```python
from build123d import *

# Parameters (mm, degrees)
SKETCH_W        = 40
SKETCH_H        = 40
PAD_DEPTH       = 37
SKETCH001_R     = 10.5
POCKET_DEPTH    = 40.001
SKETCH002_R     = 11.1
POCKET001_DEPTH = 40.001
CHAMFER_SIZE    = 2
FILLET_R        = 3
FILLET001_R     = 1


with BuildPart() as part:
    # Sketch → Pad (new body)
    with BuildSketch(Plane.XY):
        Rectangle(SKETCH_W, SKETCH_H)
    extrude(amount=PAD_DEPTH)

    # Sketch001 → Pocket (cut, through all)
    with BuildSketch(Plane.YZ.offset(20)):
        with Locations((0, 4)):
            Circle(SKETCH001_R)
    extrude(amount=-POCKET_DEPTH, mode=Mode.SUBTRACT)

    # Sketch002 → Pocket001 (cut, through all)
    with BuildSketch(Plane.XZ.offset(20)):
        with Locations((0, 30)):
            Circle(SKETCH002_R)
    extrude(amount=-POCKET001_DEPTH, mode=Mode.SUBTRACT)

    # Chamfer
    chamfer_edges = [part.edges().sort_by_distance(p)[0] for p in [
        (-20, -14.854122, 0),
        (-20, -2.038803, 14.300159),
        (-20, 10.300159, 1.961197),
        (-20, 14.854122, 0),
        (-20, 20, 18.5),
        (-20, 0, 37),
        (-20, -20, 18.5),
        (0, -20, 0),
        (-14.307261, -20, 37),
        (-3.714081, -20, 19.539809),
        (10.460191, -20, 33.714081),
        (14.307261, -20, 37),
        (20, -20, 18.5),
        (20, 14.854122, 0),
        (20, 10.300159, 1.961197),
        (20, -2.038803, 14.300159),
        (20, -14.854122, 0),
        (20, 0, 37),
        (20, 20, 18.5),
        (0, 20, 0),
        (14.307261, 20, 37),
        (10.460191, 20, 33.714081),
        (-3.714081, 20, 19.539809),
        (-14.307261, 20, 37),
    ]]
    chamfer(chamfer_edges, length=CHAMFER_SIZE)

    # Fillet
    fillet_edges = [part.edges().sort_by_distance(p)[0] for p in [
        (-8.614523, 0, 37),
        (8.614523, 0, 37),
    ]]
    fillet(fillet_edges, radius=FILLET_R)

    # Fillet001
    fillet001_edges = [part.edges().sort_by_distance(p)[0] for p in [
        (0, 9.708244, 0),
        (0, -9.708244, 0),
    ]]
    fillet(fillet001_edges, radius=FILLET001_R)


solid = part.part
```
The listing builds one solid part. Answer for the finished solid, in the listing's coordinates (mm). Coordinates: 2 decimals unless noted, no trailing zeros. Write each loop counter-clockwise with the first axis right and the second up, starting at its lowest first coordinate (ties: lowest second). Pieces come first, ordered by that corner, then holes. Notation, with made-up numbers: M -10.5,12.25 L 37.5,12.25 A33 cw 37.5,48.25 Z; hole C 73,69 d7. An arc over 180 degrees is marked long. Use a Markdown table: item, result. Add a question column.
1. Section D-D (x = 15.5) is taken. Give the vertices of the cut face in (y, z).
2. For a pull along Z with two mould halves and no side action, classify faces 1 (the flat face through (19, 15, 1)), 2 (the cylindrical face through (-0.289, -0.252, 18.904)), 3 (the conical face through (-18.319, 0.289, 14.815)), 4 (the flat face through (19, 0, 36)) as +Z half, -Z half, draft (parallel to the pull), parting line (faces both ways), or undercut.
3. Section B-B (z = 30) is taken. Give the vertices of the cut face in (x, y), plus the area to 3 significant figures.
4. Section A-A (z = 4) is taken. Give the vertices of the cut face in (x, y).
5. Given P1, Ø5, axis at x = -4, y = 12.5, coming from the +Z side; P2, Ø20, axis at x = 0, z = 30, coming from the -Y side; P3, Ø10, axis at y = 4.5, z = 12.5, coming from the -X side; P4, Ø3, axis at x = 12.5, y = 0.5, coming from the -Z side, each flat-ended and moving along its own axis, determine where each tip first touches the part or whether it passes through.
6. Straight lines are drawn through the part: line 1 along Y through (x, z) = (8, 4); line 2 along X through (y, z) = (4, 30); line 3 along X through (y, z) = (-4.5, 24). For each, find the intervals that lie inside material, in ascending order. Write a range as [from, to].
7. Section C-C (y = 0) is taken. Give the vertices of the cut face in (x, z), plus the area to 3 significant figures.
Data:
| question | item | result |
|---|---|---|
| 1 | outline | M -20,2 L -18,0 L -11.1,0 A1 ccw -10.14,1.26 A10.5 cw long 10.14,1.26 A1 ccw 11.1,0 L 18,0 L 20,2 L 20,35 L 18,37 L -18,37 L -20,35 Z |
| 2 | face 1 | -Z half |
| 2 | face 2 | undercut |
| 2 | face 3 | undercut |
| 2 | face 4 | +Z half |
| 3 | outline | M -20,-18 L -18,-20 L -13.1,-20 L -11.1,-18 L -11.1,18 L -13.1,20 L -18,20 L -20,18 Z; M 11.1,-18 L 13.1,-20 L 18,-20 L 20,-18 L 20,18 L 18,20 L 13.1,20 L 11.1,18 Z |
| 3 | area | 696 mm2 |
| 4 | outline | M -20,-18 L -18,-20 L 18,-20 L 20,-18 L 20,-12.5 L 18,-10.5 L -18,-10.5 L -20,-12.5 Z; M -20,12.5 L -18,10.5 L 18,10.5 L 20,12.5 L 20,18 L 18,20 L -18,20 L -20,18 Z |
| 5 | P1 | stops at z = 21 |
| 5 | P2 | passes through |
| 5 | P3 | stops at x = -20 |
| 5 | P4 | stops at z = 14.31 |
| 6 | line 1 | y = [-20, -10.5], [10.5, 20] |
| 6 | line 2 | x = [-20, -11.1], [11.1, 20] |
| 6 | line 3 | x = [-20, -9.34], [9.34, 20] |
| 7 | outline | M -20,16.5 L -18,14.5 L 18,14.5 L 20,16.5 L 20,35 L 18,37 L 13.52,37 A3 ccw 10.64,33.15 A11.1 cw long -10.64,33.15 A3 ccw -13.52,37 L -18,37 L -20,35 Z |
| 7 | area | 545 mm2 |
